CAD build for the part. Positions are in the model's coordinates, mm. Give positions to 0.01 mm unless a question says otherwise; leave off trailing zeros. Loops run counter-clockwise (first coordinate to the right, second up) from the corner with the lowest first, then second, coordinate; pieces in that order, holes last. Notation, with made-up numbers: M 61,56 L 93,56 A12 cw 93,76 Z; hole C -16.5,44 d3. An arc over 180 degrees is marked long. Answer as CSV lines item,"result".
from build123d import *

# Parameters (mm, degrees)
F1_DEPTH = 3.175
F2_R     = 1.27


with BuildPart() as f1:
    # F0 (on Right) → F1 (new body)
    with BuildSketch(Plane.YZ):
        with BuildLine():
            Line((-0.448989, 0), (0, 0))
            Line((0, 0), (0, 3.175))
            ThreePointArc((0, 3.175), (-4.438789, 7.408333), (0, 11.641667))
            Line((0, 11.641667), (0, 14.816667))
            Line((0, 14.816667), (-0.448989, 14.816667))
            ThreePointArc((-0.448989, 14.816667), (-4.939117, 12.956795), (-6.798989, 8.466667))
            Line((-6.798989, 8.466667), (-6.798989, 6.35))
            ThreePointArc((-6.798989, 6.35), (-4.939117, 1.859872), (-0.448989, 0))
        make_face()
    extrude(amount=F1_DEPTH)

    # F2
    f2_edges = [f1.edges().sort_by_distance(p)[0] for p in [
        (3.175, -4.438789, 7.408333),
        (0, -4.438789, 7.408333),
    ]]
    fillet(f2_edges, radius=F2_R)


solid = f1.part
1) Flat gauge pins, fed straight in: pin 1 (1.5 mm diameter, centred on x = 1.5, z = 9.5, fed in from +Y); pin 2 (1.5 mm diameter, centred on x = 0.5, z = 9.5, fed in from +Y). Where does each tip first touch, or does it go through?
Answer below:
pin 1,"stops at y = -3.34"
pin 2,"stops at y = -3.51"
2) Band-saw the part on C-C on z = 14. Give the cut face in (x, y) (3 decimals), and give its area (3 significant figures).
Answer below:
outline,"M 0,-3.564 L 3.175,-3.564 L 3.175,0 L 0,0 Z"
area,"11.3 mm^2"
3) Mould opens along Z. For faces 1 (the face through (1.583, -4.438, 7.312)), 2 (the face through (3.175, -6, 7)), 3 (the face through (1.565, -4.889, 13.006)) say: +Z half, -Z half, draft (parallel to the pull), parting line (faces both ways), or undercut.
Answer below:
face 1,"undercut"
face 2,"draft"
face 3,"+Z half"
4) Band-saw the part on D-D on z = 1.5. Give the cut face in (x, y) (3 decimals), and give its area (3 significant figures).
Answer below:
outline,"M 0,-4.548 L 3.175,-4.548 L 3.175,0 L 0,0 Z"
area,"14.4 mm^2"
5) Band-saw the part on A-A on x = 1.65. Give the cut face in (y, z) (3 decimals), and give its area (3 significant figures).
Answer below:
outline,"M -6.799,6.35 A6.35 ccw -0.449,0 L 0,0 L 0,3.175 A4.238 cw long 0,11.642 L 0,14.817 L -0.449,14.817 A6.35 ccw -6.799,8.467 Z"
area,"53.5 mm^2"
6) Drill centre lines: line 1 (Z direction, x = 2.15, y = -0.5); line 2 (Z direction, x = 2.25, y = -3.75); line 3 (Y direction, x = 1.15, z = 7.25). Where is each one in solid material? Low to high. Write a range as from..to.
Answer below:
line 1,"z = 0..3.16, 11.66..14.82"
line 2,"z = 0.93..5.01, 9.81..13.89"
line 3,"y = -6.8..-4.44"
